```python
from build123d import *

# Parameters (mm, degrees)
BOSS_EXTRUDE2_DEPTH = 5
CUT_EXTRUDE2_DEPTH  = 4
BOSS_EXTRUDE4_START = 1.2
BOSS_EXTRUDE4_DEPTH = 1.2
CUT_EXTRUDE5_DEPTH  = 1
SKETCH13_R          = 1
CUT_EXTRUDE6_DEPTH  = 58.948522414
CUT_EXTRUDE10_DEPTH = 3.7


with BuildPart() as part:
    # Sketch5 → Boss-Extrude2 (new body)
    with BuildSketch(Plane(origin=(0, 0, 0), x_dir=(1, 0, 0), z_dir=(0, 1, 0))):
        with BuildLine():
            Line((-44.375, -30.875), (41.875, -30.875))
            ThreePointArc((41.875, -30.875), (46.824747468, -28.824747468), (48.875, -23.875))
            Line((48.875, -23.875), (48.875, 26.375))
            ThreePointArc((48.875, 26.375), (47.556980515, 29.556980515), (44.375, 30.875))
            Line((44.375, 30.875), (-44.375, 30.875))
            ThreePointArc((-44.375, 30.875), (-47.556980515, 29.556980515), (-48.875, 26.375))
            Line((-48.875, 26.375), (-48.875, -26.375))
            ThreePointArc((-48.875, -26.375), (-47.556980515, -29.556980515), (-44.375, -30.875))
        make_face()
    extrude(amount=BOSS_EXTRUDE2_DEPTH)

    # Sketch10 → Cut-Extrude2 (cut)
    with BuildSketch(Plane.XZ):
        with BuildLine():
            Line((-48.875, 18), (-44.460786438, 13.585786438))
            ThreePointArc((-44.460786438, 13.585786438), (-44.027240935, 12.93693974), (-43.875, 12.171572875))
            Line((-43.875, 12.171572875), (-43.875, -12.171572875))
            ThreePointArc((-43.875, -12.171572875), (-44.027240935, -12.93693974), (-44.460786438, -13.585786438))
            Line((-44.460786438, -13.585786438), (-48.875, -18))
            Line((-48.875, -18), (-48.875, 18))
        make_face()
        with BuildLine():
            Line((48.875, -18), (48.875, 18))
            Line((48.875, 18), (44.460786438, 13.585786438))
            ThreePointArc((44.460786438, 13.585786438), (44.027240935, 12.93693974), (43.875, 12.171572875))
            Line((43.875, 12.171572875), (43.875, -12.171572875))
            ThreePointArc((43.875, -12.171572875), (44.027240935, -12.93693974), (44.460786438, -13.585786438))
            Line((44.460786438, -13.585786438), (48.875, -18))
        make_face()
        with BuildLine():
            Line((-38, -30.875), (-35.585786438, -28.460786438))
            ThreePointArc((-35.585786438, -28.460786438), (-34.93693974, -28.027240935), (-34.171572875, -27.875))
            Line((-34.171572875, -27.875), (34.171572875, -27.875))
            ThreePointArc((34.171572875, -27.875), (34.93693974, -28.027240935), (35.585786438, -28.460786438))
            Line((35.585786438, -28.460786438), (38, -30.875))
            Line((38, -30.875), (-38, -30.875))
        make_face()
        with BuildLine():
            Line((-38, 30.875), (38, 30.875))
            Line((38, 30.875), (35.585786438, 28.460786438))
            ThreePointArc((35.585786438, 28.460786438), (34.93693974, 28.027240935), (34.171572875, 27.875))
            Line((34.171572875, 27.875), (-34.171572875, 27.875))
            ThreePointArc((-34.171572875, 27.875), (-34.93693974, 28.027240935), (-35.585786438, 28.460786438))
            Line((-35.585786438, 28.460786438), (-38, 30.875))
        make_face()
    extrude(amount=-CUT_EXTRUDE2_DEPTH, mode=Mode.SUBTRACT)

    # Sketch11 → Boss-Extrude4 (add)
    with BuildSketch(Plane.XZ.offset(-4).offset(BOSS_EXTRUDE4_START)):
        with BuildLine():
            Line((-35.585786438, -28.460786438), (-36.5, -29.375))
            Line((-36.5, -29.375), (36.5, -29.375))
            Line((36.5, -29.375), (35.585786438, -28.460786438))
            ThreePointArc((35.585786438, -28.460786438), (34.93693974, -28.027240935), (34.171572875, -27.875))
            Line((34.171572875, -27.875), (-34.171572875, -27.875))
            ThreePointArc((-34.171572875, -27.875), (-34.93693974, -28.027240935), (-35.585786438, -28.460786438))
        make_face()
        with BuildLine():
            Line((-36.5, 29.375), (-35.585786438, 28.460786438))
            ThreePointArc((-35.585786438, 28.460786438), (-34.93693974, 28.027240935), (-34.171572875, 27.875))
            Line((-34.171572875, 27.875), (34.171572875, 27.875))
            ThreePointArc((34.171572875, 27.875), (34.93693974, 28.027240935), (35.585786438, 28.460786438))
            Line((35.585786438, 28.460786438), (36.5, 29.375))
            Line((36.5, 29.375), (-36.5, 29.375))
        make_face()
    extrude(amount=-BOSS_EXTRUDE4_DEPTH)

    # Sketch6 → Cut-Extrude5 (cut)
    with BuildSketch(Plane.XZ):
        with BuildLine():
            Line((-47.975, 26.375), (-47.975, 19.975))
            ThreePointArc((-47.975, 19.975), (-47.345745068, 18.753606113), (-45.985929297, 18.55696973))
            Line((-45.985929297, 18.55696973), (-39.985929297, 20.626336144))
            ThreePointArc((-39.985929297, 20.626336144), (-39.253606113, 21.173621347), (-38.975, 22.044366415))
            Line((-38.975, 22.044366415), (-38.975, 28.475))
            ThreePointArc((-38.975, 28.475), (-39.414339828, 29.535660172), (-40.475, 29.975))
            Line((-40.475, 29.975), (-44.375, 29.975))
            ThreePointArc((-44.375, 29.975), (-46.920584412, 28.920584412), (-47.975, 26.375))
        make_face()
        with BuildLine():
            Line((40.475, 29.975), (41.875, 29.975))
            ThreePointArc((41.875, 29.975), (46.188351365, 28.188351365), (47.975, 23.875))
            Line((47.975, 23.875), (47.975, 19.975))
            ThreePointArc((47.975, 19.975), (47.345745068, 18.753606113), (45.985929297, 18.55696973))
            Line((45.985929297, 18.55696973), (39.985929297, 20.626336144))
            ThreePointArc((39.985929297, 20.626336144), (39.253606113, 21.173621347), (38.975, 22.044366415))
            Line((38.975, 22.044366415), (38.975, 28.475))
            ThreePointArc((38.975, 28.475), (39.414339828, 29.535660172), (40.475, 29.975))
        make_face()
        with BuildLine():
            Line((47.975, -26.375), (47.975, -19.975))
            ThreePointArc((47.975, -19.975), (47.345745068, -18.753606113), (45.985929297, -18.55696973))
            Line((45.985929297, -18.55696973), (39.985929297, -20.626336144))
            ThreePointArc((39.985929297, -20.626336144), (39.253606113, -21.173621347), (38.975, -22.044366415))
            Line((38.975, -22.044366415), (38.975, -28.475))
            ThreePointArc((38.975, -28.475), (39.414339828, -29.535660172), (40.475, -29.975))
            Line((40.475, -29.975), (44.375, -29.975))
            ThreePointArc((44.375, -29.975), (46.920584412, -28.920584412), (47.975, -26.375))
        make_face()
        with BuildLine():
            Line((-40.475, -29.975), (-44.375, -29.975))
            ThreePointArc((-44.375, -29.975), (-46.920584412, -28.920584412), (-47.975, -26.375))
            Line((-47.975, -26.375), (-47.975, -19.975))
            ThreePointArc((-47.975, -19.975), (-47.345745068, -18.753606113), (-45.985929297, -18.55696973))
            Line((-45.985929297, -18.55696973), (-39.985929297, -20.626336144))
            ThreePointArc((-39.985929297, -20.626336144), (-39.253606113, -21.173621347), (-38.975, -22.044366415))
            Line((-38.975, -22.044366415), (-38.975, -28.475))
            ThreePointArc((-38.975, -28.475), (-39.414339828, -29.535660172), (-40.475, -29.975))
        make_face()
    extrude(amount=-CUT_EXTRUDE5_DEPTH, mode=Mode.SUBTRACT)

    # Sketch13 → Cut-Extrude6 (cut, through all)
    with BuildSketch(Plane.XZ.offset(-1)):
        with Locations(Location((-45, 27.04, 0), (0, 0, 270))):
            Circle(SKETCH13_R)
        with Locations(Location((-45, -27.04, 0), (0, 0, 90))):
            Circle(SKETCH13_R)
        with Locations(Location((45, -27.04, 0), (0, 0, 270))):
            Circle(SKETCH13_R)
        with Locations(Location((45, 24, 0), (0, 0, 270))):
            Circle(SKETCH13_R)
    extrude(amount=-CUT_EXTRUDE6_DEPTH, mode=Mode.SUBTRACT)

    # Sketch16 → Cut-Extrude10 (cut)
    with BuildSketch(Plane(origin=(0, 5, 0), x_dir=(1, 0, 0), z_dir=(0, 1, 0))):
        with BuildLine():
            Line((-37.275, 27.275), (37.275, 27.275))
            ThreePointArc((37.275, 27.275), (41.517640687, 25.517640687), (43.275, 21.275))
            Line((43.275, 21.275), (43.275, -21.275))
            ThreePointArc((43.275, -21.275), (41.517640687, -25.517640687), (37.275, -27.275))
            Line((37.275, -27.275), (-37.275, -27.275))
            ThreePointArc((-37.275, -27.275), (-41.517640687, -25.517640687), (-43.275, -21.275))
            Line((-43.275, -21.275), (-43.275, 21.275))
            ThreePointArc((-43.275, 21.275), (-41.517640687, 25.517640687), (-37.275, 27.275))
        make_face()
    extrude(amount=-CUT_EXTRUDE10_DEPTH, mode=Mode.SUBTRACT)


solid = part.part
```
CAD build for the part. Positions are in the model's coordinates, mm. A direction names the side the tool comes from. Coordinates: 2 decimals unless noted, no trailing zeros. Write each loop counter-clockwise with the first axis right and the second up, starting at its lowest first coordinate (ties: lowest second). Pieces come first, ordered by that corner, then holes.
(1) 3-axis set-ups, long thin cutter, end or side, ignore diameter. For faces 5 (the face through (-43.028, 0.493, -19.577)), 6 (the face through (46, 4, 0)), 7 (the face through (-46, 4, 0)): which of +Z, -Z, +X, -X, +Y, -Y reach the whole face in a straight line?
(2) Flat gauge pins, fed straight in: pin 1 (2 mm diameter, centred on y = 2.5, z = 0.5, fed in from -X) (3 decimals); pin 2 (4 mm diameter, centred on x = -29.5, z = 12.5, fed in from +Y); pin 3 (1.5 mm diameter, centred on x = 47, z = -9, fed in from -Y). Where does each tip first touch, or does it go through?
(3) Drill centre lines: probe 1 along Z at (x, y) = (28.5, 4.35) (3 decimals); probe 2 along X at (y, z) = (4.15, 21.5) (3 decimals); probe 3 along X at (y, z) = (2.35, -8) (3 decimals). Where is each one in solid material? Low to high.
(4) Two-plate mould, pull along X, no slides. Class faces 1 (the face through (43.875, 2, 0)), 2 (the face through (-41.471, 3.176, 25.564)), 3 (the face through (-4.6, 4.3, 30.875)), 4 (the face through (-36.81, 1.972, -29.685)): +X half, -X half, draft (parallel to the pull), parting line (faces both ways), or undercut.
(5) Cut at A-A, the plane x = 9.5. List the corners of the cut face in (y, z) (3 decimals).
(6) Cut at B-B, the plane z = -5. List the corners of the cut face in (x, y) (3 decimals).
Geometry says:
1. face 5: -Y
1. face 6: +X, -Y
1. face 7: -X, -Y
2. pin 1: stops at x = -43.875
2. pin 2: stops at y = 1.3
2. pin 3: stops at y = 4
3. probe 1: z = -30.875 to -27.275, 27.275 to 30.875
3. probe 2: x = -48.875 to -43.271, 43.271 to 48.875
3. probe 3: x = -43.875 to -43.275, 43.275 to 43.875
4. face 1: +X half
4. face 2: undercut
4. face 3: draft
4. face 4: undercut
5. outline: (0, -27.875) - (2.8, -27.875) - (2.8, -29.375) - (4, -29.375) - (4, -30.875) - (5, -30.875) - (5, -27.275) - (1.3, -27.275) - (1.3, 27.275) - (5, 27.275) - (5, 30.875) - (4, 30.875) - (4, 29.375) - (2.8, 29.375) - (2.8, 27.875) - (0, 27.875) - close
6. outline: (-48.875, 4) - (-43.875, 4) - (-43.875, 0) - (43.875, 0) - (43.875, 4) - (48.875, 4) - (48.875, 5) - (43.275, 5) - (43.275, 1.3) - (-43.275, 1.3) - (-43.275, 5) - (-48.875, 5) - close
